```python
from build123d import *

# Parameters (mm, degrees)
F1_DEPTH       = 18
F2_R           = 7.5
F3_DEPTH       = 46.001
F5_D           = 10
F5_CBORE_D     = 17
F5_CBORE_DEPTH = 10
F6_SIZE2       = 1
F6_SIZE        = 1
F7_R           = 0.5


with BuildPart() as f1:
    # F0 (on Front) → F1 (new body, symmetric)
    with BuildSketch(Plane.XZ):
        with BuildLine():
            ThreePointArc((30, 21), (29.4142135624, 22.4142135624), (28, 23))
            Line((28, 23), (-15, 23))
            ThreePointArc((-15, 23), (-22.0710678119, 20.0710678119), (-25, 13))
            Line((-25, 13), (-30, 8))
            Line((-30, 8), (-30, -8))
            Line((-30, -8), (-25, -13))
            ThreePointArc((-25, -13), (-22.0710678119, -20.0710678119), (-15, -23))
            Line((-15, -23), (28, -23))
            ThreePointArc((28, -23), (29.4142135624, -22.4142135624), (30, -21))
            Line((30, -21), (30, -17))
            ThreePointArc((30, -17), (29.4142135624, -15.5857864376), (28, -15))
            Line((28, -15), (-11, -15))
            ThreePointArc((-11, -15), (-13.8284271247, -13.8284271247), (-15, -11))
            Line((-15, -11), (-15, 11))
            ThreePointArc((-15, 11), (-13.8284271247, 13.8284271247), (-11, 15))
            Line((-11, 15), (28, 15))
            ThreePointArc((28, 15), (29.4142135624, 15.5857864376), (30, 17))
            Line((30, 17), (30, 21))
        make_face()
    extrude(amount=F1_DEPTH, both=True)

    # F2 (on face) → F3 (cut, through all)
    with BuildSketch(Plane.XY.offset(23)):
        with Locations((18, 0)):
            Circle(F2_R)
    extrude(amount=-F3_DEPTH, mode=Mode.SUBTRACT)

    # F5 (through all)
    with Locations(Plane.YZ.offset(-15)):
        with Locations((0, 0)):
            CounterBoreHole(F5_D / 2, F5_CBORE_D / 2, F5_CBORE_DEPTH)

    # F6
    f6_edges = [f1.edges().sort_by_distance(p)[0] for p in [
        (10.5, 0, -23),
        (10.5, 0, 23),
        (-30, -5, 0),
    ]]
    chamfer(f6_edges, length=F6_SIZE, length2=F6_SIZE2)

    # F7
    f7_edges = [f1.edges().sort_by_distance(p)[0] for p in [
        (29.414214, 18, 22.414214),
        (6.5, 18, 23),
        (-22.071068, 18, 20.071068),
        (-27.5, 18, 10.5),
        (-30, 18, 0),
        (-27.5, 18, -10.5),
        (-22.071068, 18, -20.071068),
        (6.5, 18, -23),
        (29.414214, 18, -22.414214),
        (30, 18, -19),
        (29.414214, 18, -15.585786),
        (8.5, 18, -15),
        (-13.828427, 18, -13.828427),
        (-15, 18, 0),
        (-13.828427, 18, 13.828427),
        (8.5, 18, 15),
        (29.414214, 18, 15.585786),
        (30, 18, 19),
        (29.414214, -18, 22.414214),
        (6.5, -18, 23),
        (-22.071068, -18, 20.071068),
        (-27.5, -18, 10.5),
        (-30, -18, 0),
        (-27.5, -18, -10.5),
        (-22.071068, -18, -20.071068),
        (6.5, -18, -23),
        (29.414214, -18, -22.414214),
        (30, -18, -19),
        (29.414214, -18, -15.585786),
        (8.5, -18, -15),
        (-13.828427, -18, -13.828427),
        (-15, -18, 0),
        (-13.828427, -18, 13.828427),
        (8.5, -18, 15),
        (29.414214, -18, 15.585786),
        (30, -18, 19),
    ]]
    fillet(f7_edges, radius=F7_R)


solid = f1.part
```
Input: part model. Units: mm. Frame: model coordinates. A direction names the side the tool comes from. Coordinates: 2 decimals unless noted, no trailing zeros. Loops run counter-clockwise (first coordinate to the right, second up) from the corner with the lowest first, then second, coordinate; pieces in that order, holes last. Notation, with made-up numbers: M -5.75,27 L 2.25,27 A24 ccw 2.25,49 Z; hole C -37,85 d10. An arc over 180 degrees is marked long. Use a Markdown table: item, result. Add a question column.
1) Pin query (flat end, axial travel): P1, Ø5, axis at y = 5.5, z = 9, coming from the +X side; P2, Ø6, axis at x = -16.5, y = -11, coming from the +Z side; P3, Ø1.5, axis at y = -13, z = 17, coming from the -X side; P4, Ø9, axis at x = 18, y = 0, coming from the +Z side. Return the tip coordinate at first contact, or that it passes through.
2) Section D-D, the plane y = -10. Return the cut outline in (x, z), plus the area to 3 significant figures.
3) Section B-B, the plane z = 0. Return the cut outline in (x, y), plus the area to 3 significant figures.
4) Line query: L1, parallel to Z at x = -6.5, y = 11.5; L2, parallel to X at y = 9, z = -6.5; L3, parallel to Y at x = 18, z = -20. Output: solid intervals per line, ascending. Write a range as from..to.
5) Set-up query: faces 1 (the flat face through (-15, -8, -5)), 2 (the cylindrical face through (-19.93, 4.57, 7.167)), 3 (the flat face through (-18, 18, 0)). Return all of +Z, -Z, +X, -X, +Y, -Y with unobstructed straight access to the full face (end or side cutting, diameter ignored); none if empty.
6) Draft query along Z for faces 4 (the cylindrical face through (-22.15, -0.25, -19.99)), 5 (the flat face through (9, 0, -15)), 6 (the cylindrical face through (10.507, 0.33, 18.549)), 7 (the flat face through (8, 0, 15)). Return one class per face: +Z half, -Z half, draft (parallel to the pull), parting line (faces both ways), or undercut.
7) Section A-A, the plane x = 1. Return the cut outline in (y, z).
8) Section C-C, the plane x = 18. Return the cut outline in (y, z), plus the area to 3 significant figures.
Answer below:
| question | item | result |
|---|---|---|
| 1 | P1 | x = -14.97 |
| 1 | P2 | z = 23 |
| 1 | P3 | x = -24.46 |
| 1 | P4 | through |
| 2 | outline | M -30,-8 L -25,-13 A10 ccw -15,-23 L 28,-23 A2 ccw 30,-21 L 30,-17 A2 ccw 28,-15 L -11,-15 A4 cw -15,-11 L -15,11 A4 cw -11,15 L 28,15 A2 ccw 30,17 L 30,21 A2 ccw 28,23 L -15,23 A10 ccw -25,13 L -30,8 Z |
| 2 | area | 1,250 mm2 |
| 3 | outline | M -30,-17.5 A0.5 ccw -29.5,-18 L -15.5,-18 A0.5 ccw -15,-17.5 L -15,-8.5 L -25,-8.5 L -25,-5 L -29,-5 L -30,-6 Z; M -30,6 L -29,5 L -25,5 L -25,8.5 L -15,8.5 L -15,17.5 A0.5 ccw -15.5,18 L -29.5,18 A0.5 ccw -30,17.5 Z |
| 3 | area | 319 mm2 |
| 4 | L1 | -23..-15, 15..23 |
| 4 | L2 | -30..-15 |
| 4 | L3 | -18..-7.5, 7.5..18 |
| 5 | face 1 | +X, +Y, -Y |
| 5 | face 2 | +X |
| 5 | face 3 | +Z, -Z, +X, -X, +Y |
| 6 | face 4 | -Z half |
| 6 | face 5 | undercut |
| 6 | face 6 | draft |
| 6 | face 7 | undercut |
| 7 | outline | M -18,-22.5 A0.5 ccw -17.5,-23 L 17.5,-23 A0.5 ccw 18,-22.5 L 18,-15.5 A0.5 ccw 17.5,-15 L -17.5,-15 A0.5 ccw -18,-15.5 Z; M -18,15.5 A0.5 ccw -17.5,15 L 17.5,15 A0.5 ccw 18,15.5 L 18,22.5 A0.5 ccw 17.5,23 L -17.5,23 A0.5 ccw -18,22.5 Z |
| 8 | outline | M -18,-22.5 A0.5 ccw -17.5,-23 L -8.5,-23 L -7.5,-22 L -7.5,-15 L -17.5,-15 A0.5 ccw -18,-15.5 Z; M -18,15.5 A0.5 ccw -17.5,15 L -7.5,15 L -7.5,22 L -8.5,23 L -17.5,23 A0.5 ccw -18,22.5 Z; M 7.5,-22 L 8.5,-23 L 17.5,-23 A0.5 ccw 18,-22.5 L 18,-15.5 A0.5 ccw 17.5,-15 L 7.5,-15 Z; M 7.5,15 L 17.5,15 A0.5 ccw 18,15.5 L 18,22.5 A0.5 ccw 17.5,23 L 8.5,23 L 7.5,22 Z |
| 8 | area | 334 mm2 |
